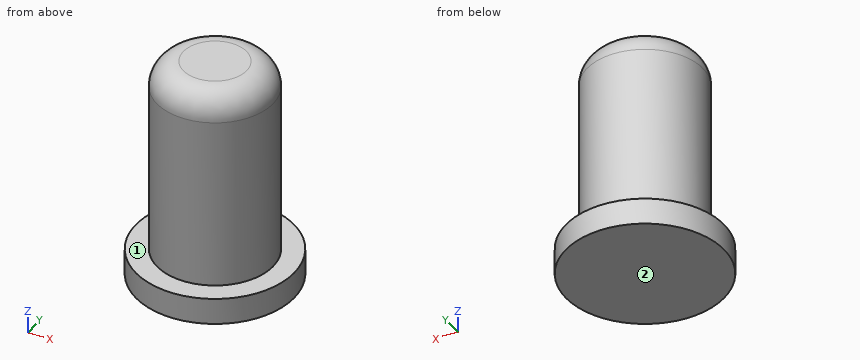
```python
from build123d import *

# Parameters (mm, degrees)
CYLINDER020_R     = 2.2
CYLINDER020_DEPTH = 8.5
CYLINDER022_R     = 3
CYLINDER022_DEPTH = 1
FILLET001_R       = 1


with BuildPart() as control_button_c:
    # Cylinder020 → Cylinder020 (new body)
    with BuildSketch(Plane(origin=(58.3, 98.3, 9.6), x_dir=(1, 0, 0), z_dir=(0, 0, 1))):
        Circle(CYLINDER020_R)
    extrude(amount=CYLINDER020_DEPTH)


with BuildPart() as control_button:
    # Cylinder022 → Cylinder022 (new body)
    with BuildSketch(Plane(origin=(58.3, 98.3, 9.6), x_dir=(1, 0, 0), z_dir=(0, 0, 1))):
        Circle(CYLINDER022_R)
    extrude(amount=CYLINDER022_DEPTH)

    # Fusion033: union control_button_c
    add(control_button_c.part)

    # Fillet001
    fillet001_edges = [control_button.edges().sort_by_distance(p)[0] for p in [
        (56.1, 98.3, 18.1),
    ]]
    fillet(fillet001_edges, radius=FILLET001_R)


solid = control_button.part
```
Design review of the part built by this model. Coordinates are the model's own, in mm. Face numbers are marked on the shaded views. A direction names the side the tool comes from. Round coordinates to 2 decimals unless told otherwise and drop trailing zeros. Write each loop counter-clockwise with the first axis right and the second up, starting at its lowest first coordinate (ties: lowest second). Pieces come first, ordered by that corner, then holes. Notation, with made-up numbers: (9.5, -1) -> (34.5, -1) arc R10 cw to (34.5, 8) -> close; hole circle Ø1 at (-11.75, 86). An arc over 180 degrees is marked (long way). Answer in a Markdown table with one row per item.
Q1. For the marked faces 1 and 2, list the 3-axis set-ups (+Z, -Z, +X, -X, +Y, -Y) from which the entire face can be reached by the end or side of a thin tool; tool diameter is ignored.
The answers:
| item | result |
|---|---|
| face 1 | +Z |
| face 2 | -Z, +X, -X, +Y, -Y |
Q2. To check wall thickness, follow L1, parallel to Z at x = 58.3, y = 99.55; L2, parallel to X at y = 98.2, z = 11.5; L3, parallel to Z at x = 56.35, y = 99.9. State the ranges of each line that lie inside material, in increasing order. Write a range as [from, to].
The answers:
| item | result |
|---|---|
| L1 | [9.6, 18.1] |
| L2 | [56.1, 60.5] |
| L3 | [9.6, 10.6] |
Q3. Take a section at B-B, the plane x = 58.3. State the section outline as (y, z) points, then the cut area to 3 significant figures.
The answers:
| item | result |
|---|---|
| outline | (95.3, 9.6) -> (101.3, 9.6) -> (101.3, 10.6) -> (100.5, 10.6) -> (100.5, 17.1) arc R1 ccw to (99.5, 18.1) -> (97.1, 18.1) arc R1 ccw to (96.1, 17.1) -> (96.1, 10.6) -> (95.3, 10.6) -> close |
| area | 38.6 mm² |
Q4. Take a section at D-D, the plane x = 60.75. State the section outline as (y, z) points.
The answers:
| item | result |
|---|---|
| outline | (96.57, 9.6) -> (100.03, 9.6) -> (100.03, 10.6) -> (96.57, 10.6) -> close |
Q5. Clearance check with flat-ended pins moving along their axes: pin 1 Ø1.5 at (y, z) = (98, 16.5) entering from -X; pin 2 Ø2 at (x, z) = (58, 14) entering from -Y. State where each tip first meets the part, or that it passes through.
The answers:
| item | result |
|---|---|
| pin 1 | x = 56.1 |
| pin 2 | y = 96.1 |
Q6. Take a section at C-C, the plane z = 13.75. State the section outline as (x, y) points.
The answers:
| item | result |
|---|---|
| outline | circle Ø4.4 at (58.3, 98.3) |
Q7. Take a section at A-A, the plane y = 98.3. State the section outline as (x, z) points.
The answers:
| item | result |
|---|---|
| outline | (55.3, 9.6) -> (61.3, 9.6) -> (61.3, 10.6) -> (60.5, 10.6) -> (60.5, 17.1) arc R1 ccw to (59.5, 18.1) -> (57.1, 18.1) arc R1 ccw to (56.1, 17.1) -> (56.1, 10.6) -> (55.3, 10.6) -> close |
